Geometry: final body of the model. Coordinates: model frame, mm. A direction names the side the tool comes from. Give positions to 0.01 mm unless a question says otherwise; leave off trailing zeros. Order: outer loops, then holes, each group sorted by start corner. A loop starts at its lowest first (then second) coordinate and runs counter-clockwise, first axis right, second up. Notation, with made-up numbers: (3.5, 59.25) -> (51.5, 59.25) arc R25 ccw to (51.5, 89.25) -> close; hole circle Ø7 at (-21.75, -36). An arc over 180 degrees is marked (long way). One line per question, with ' | ' between items.
from build123d import *

# Parameters (mm, degrees)
F0_R     = 203.2
F1_DEPTH = 6.35
F3_DEPTH = 6.351
F5_DEPTH = 6.351
F6_R     = 19.05
F7_DEPTH = 6.351


with BuildPart() as f1:
    # F0 (on Top) → F1 (new body)
    with BuildSketch(Plane.XY):
        Circle(F0_R)
    extrude(amount=F1_DEPTH)

    # F2 (on face) → F3 (cut, through all)
    with BuildSketch(Plane.XY.offset(6.35)):
        with BuildLine():
            ThreePointArc((-200.704204, 31.75), (-203.2, 0), (-200.704204, -31.75))
            Line((-200.704204, -31.75), (-137.204204, -31.75))
            Line((-137.204204, -31.75), (-137.204204, 31.75))
            Line((-137.204204, 31.75), (-200.704204, 31.75))
        make_face()
    extrude(amount=-F3_DEPTH, mode=Mode.SUBTRACT)

    # F4 (on face) → F5 (cut, through all)
    with BuildSketch(Plane.XY.offset(6.35)):
        Polygon((50.8, 31.75), (50.8, -31.75), (114.3, -31.75), (188.371442, -76.2), (188.371442, 76.2), (114.3, 31.75), align=None)
        with BuildLine():
            Line((188.371442, 76.2), (188.371442, -76.2))
            ThreePointArc((188.371442, -76.2), (203.2, 0), (188.371442, 76.2))
        make_face()
    extrude(amount=-F5_DEPTH, mode=Mode.SUBTRACT)

    # F6 (on face) → F7 (cut, through all)
    with BuildSketch(Plane.XY.offset(6.35)):
        with Locations((-73.704204, 0)):
            Circle(F6_R)
    extrude(amount=-F7_DEPTH, mode=Mode.SUBTRACT)


solid = f1.part
1) Section B-B on x = 136. Return loops of the section in (y, z), plus the area to 3 significant figures.
Check result:
outline: (-150.98, 0) -> (-44.77, 0) -> (-44.77, 6.35) -> (-150.98, 6.35) -> close; (44.77, 0) -> (150.98, 0) -> (150.98, 6.35) -> (44.77, 6.35) -> close | area: 1,350 mm^2
2) Section D-D on y = 115. Return loops of the section in (x, z).
Check result:
outline: (-167.53, 0) -> (167.53, 0) -> (167.53, 6.35) -> (-167.53, 6.35) -> close
3) Section A-A on z = 1.75. Return loops of the section in (x, y).
Check result:
outline: (-200.7, -31.75) arc R203.2 ccw to (188.37, -76.2) -> (114.3, -31.75) -> (50.8, -31.75) -> (50.8, 31.75) -> (114.3, 31.75) -> (188.37, 76.2) arc R203.2 ccw to (-200.7, 31.75) -> (-137.2, 31.75) -> (-137.2, -31.75) -> close; hole circle Ø38.1 at (-73.7, 0)
4) Material intervals for probe 1 along Y at (x, z) = (127, 3); probe 2 along X at (y, z) = (171.5, 1.25); probe 3 along X at (y, z) = (38, 1) (3 decimals), sorted ascending. Write a range as from..to.
Check result:
probe 1: y = -158.62..-39.37, 39.37..158.62 | probe 2: x = -108.99..108.99 | probe 3: x = -199.615..124.715
5) Contact query for flat-ended pins moving along their axis: pin 1 Ø2 at (x, y) = (37.5, -80) entering from -Z; pin 2 Ø1 at (x, z) = (75.5, 4) entering from +Y; pin 3 Ø3 at (x, z) = (54.5, 4.5) entering from +Y; pin 4 Ø3 at (x, z) = (-139, 4) entering from +Y. Output: stop coordinate, or through.
Check result:
pin 1: stops at z = 0 | pin 2: stops at y = 188.85 | pin 3: stops at y = 196.17 | pin 4: stops at y = 149.61
6) Set-up query: faces 1 (the cylindrical face through (-55.534, 5.722, 3.219)), 2 (the flat face through (151.854, 54.286, 3.219)). Return all of +Z, -Z, +X, -X, +Y, -Y with unobstructed straight access to the full face (end or side cutting, diameter ignored); none if empty.
Check result:
face 1: +Z, -Z | face 2: +Z, -Z, +X
7) Section C-C on y = 0. Return loops of the section in (x, z), plus the area to 3 significant figures.
Check result:
outline: (-137.2, 0) -> (-92.75, 0) -> (-92.75, 6.35) -> (-137.2, 6.35) -> close; (-54.65, 0) -> (50.8, 0) -> (50.8, 6.35) -> (-54.65, 6.35) -> close | area: 952 mm^2
8) Pull-direction query (Y, two-part tool) for faces 3 (the cylindrical face through (-19.386, 202.273, 3.131)), 4 (the flat face through (150.817, -53.664, 3.219)), 5 (the flat face through (-9, 3, 6.35)); classes: +Y half, -Y half, draft (parallel to the pull), parting line (faces both ways), or undercut.
Check result:
face 3: +Y half | face 4: undercut | face 5: draft
